Part model, mm, in its own coordinate system. A direction names the side the tool comes from. Coordinates: 2 decimals unless noted, no trailing zeros. Order: outer loops, then holes, each group sorted by start corner. A loop starts at its lowest first (then second) coordinate and runs counter-clockwise, first axis right, second up.
```python
from build123d import *

# Parameters (mm, degrees)
ESQUISSE1_R        = 2
ESQUISSE1_W        = 17
ESQUISSE1_H        = 7
ESQUISSE1_W_2      = 4
ESQUISSE1_H_2      = 40
ESQUISSE1_W_3      = 5
ESQUISSE1_H_3      = 5
BOSS_EXTRU_1_DEPTH = 5
CONG_1_R           = 5


with BuildPart() as part:
    # Esquisse1 → Boss.-Extru.1 (new body)
    with BuildSketch(Plane.XY):
        Polygon((0, 37.65), (71, 37.65), (71, -37.65), (0, -37.65), (0, -25), (-35, -25), (-35, -10), (-5, -10), (-5, 10), (-35, 10), (-35, 25), (0, 25), align=None)
        with Locations((-30, 17.5)):
            Circle(ESQUISSE1_R, mode=Mode.SUBTRACT)
        with Locations(Location((-30, -17.5, 0), (0, 0, 180))):
            Circle(ESQUISSE1_R, mode=Mode.SUBTRACT)
        with Locations((36, 33.15)):
            Circle(ESQUISSE1_R, mode=Mode.SUBTRACT)
        with Locations(Location((36, -33.15, 0), (0, 0, 90))):
            Circle(ESQUISSE1_R, mode=Mode.SUBTRACT)
        with Locations((28.5, -7.15)):
            Rectangle(ESQUISSE1_W, ESQUISSE1_H, mode=Mode.SUBTRACT)
        with Locations((63, 0)):
            Rectangle(ESQUISSE1_W_2, ESQUISSE1_H_2, mode=Mode.SUBTRACT)
        with Locations((28.5, 33.15)):
            Rectangle(ESQUISSE1_W_3, ESQUISSE1_H_3, mode=Mode.SUBTRACT)
        with Locations((43.5, 33.15)):
            Rectangle(ESQUISSE1_W_3, ESQUISSE1_H_3, mode=Mode.SUBTRACT)
        with Locations((28.5, -33.15)):
            Rectangle(ESQUISSE1_W_3, ESQUISSE1_H_3, mode=Mode.SUBTRACT)
        with Locations((43.5, -33.15)):
            Rectangle(ESQUISSE1_W_3, ESQUISSE1_H_3, mode=Mode.SUBTRACT)
    extrude(amount=BOSS_EXTRU_1_DEPTH)

    # Congé1
    cong_1_edges = [part.edges().sort_by_distance(p)[0] for p in [
        (-35, -10, 2.5),
        (-35, 10, 2.5),
        (-35, 25, 2.5),
        (-35, -25, 2.5),
    ]]
    fillet(cong_1_edges, radius=CONG_1_R)


solid = part.part
```
(1) Slice it at D-D, the plane y = 17.5. Give the cut face in (x, z).
(2) Slice it at C-C, the plane z = 3.8. State how many separate pieces and enclosed holes the cut face has, then the cut area to 3 significant figures.
(3) Tool access for faces 1 (the face through (-17, 10, 2)), 2 (the face through (-35, 17, 2)), 3 (the face through (43, 35.65, 2)), 4 (the face through (0, -31, 2)), 5 (the face through (-33, 24, 3)): list every direction of +Z, -Z, +X, -X, +Y, -Y with a clear straight run to the whole face (end or side of a thin tool).
(4) Drop a flat-ended pin along its axis: pin 1 (1.5 mm diameter, centred on x = -4.5, z = 3.5, fed in from +Y). Give the stop position or say it passes through.
(5) Slice it at A-A, the plane y = -7.5. Give the cut face in (x, z).
(6) Slice it at B-B, the plane y = 1. Give the cut face in (x, z).
(7) Probe line 1 (X direction, y = -33.15, z = 2.4); line 2 (Y direction, x = 36, z = 1.2); line 3 (Y direction, x = -30, z = 2.7). List the from-to ranges inside material, lowest first.
(8) Pull direction X, two halves, no side cores. Call faces 6 (the face through (-34, -12, 3)), 7 (the face through (-15, -25, 2)), 8 (the face through (26, 33, 2)): +X half, -X half, draft (parallel to the pull), parting line (faces both ways), or undercut.
Here are the results:
1. outline: (-35, 0) - (-32, 0) - (-32, 5) - (-35, 5) - close; (-28, 0) - (61, 0) - (61, 5) - (-28, 5) - close; (65, 0) - (71, 0) - (71, 5) - (65, 5) - close
2. separate pieces: 1
2. enclosed holes: 10
2. area: 6,050 mm2
3. face 1: +Z, -Z, -X
3. face 2: +Z, -Z, -X, +Y, -Y
3. face 3: +Z, -Z
3. face 4: +Z, -Z, -X, -Y
3. face 5: +Z, -Z, -X, +Y
4. pin 1: stops at y = 25
5. outline: (-5, 0) - (20, 0) - (20, 5) - (-5, 5) - close; (37, 0) - (61, 0) - (61, 5) - (37, 5) - close; (65, 0) - (71, 0) - (71, 5) - (65, 5) - close
6. outline: (-5, 0) - (61, 0) - (61, 5) - (-5, 5) - close; (65, 0) - (71, 0) - (71, 5) - (65, 5) - close
7. line 1: x = 0 to 26, 31 to 34, 38 to 41, 46 to 71
7. line 2: y = -37.65 to -35.15, -31.15 to -10.65, -3.65 to 31.15, 35.15 to 37.65
7. line 3: y = -25 to -19.5, -15.5 to -10, 10 to 15.5, 19.5 to 25
8. face 6: -X half
8. face 7: draft
8. face 8: undercut
